Source: CAD feature listing. Evaluate the final solid. Frame: model axes, mm. A direction names the side the tool comes from. Coordinates: 2 decimals unless noted, no trailing zeros. Order: outer loops, then holes, each group sorted by start corner. A loop starts at its lowest first (then second) coordinate and runs counter-clockwise, first axis right, second up. Notation, with made-up numbers: (8.5, 27.5) -> (32.5, 27.5) arc R23 cw to (32.5, 49.5) -> close; hole circle Ø10 at (-38, 69.5). An arc over 180 degrees is marked (long way). Write item = value, one per line. Start each with the question number.
Item 1: Section query D-D (x = 8.6). Output: boundary loops of the cut face in (y, z).
Item 2: Ray query, line 1 along X through (y, z) = (3.25, -3.25); line 2 along Y through (x, z) = (3.5, 4.25); line 3 along Z through (x, y) = (5.5, 3.5). Return the intervals inside material, ascending. Write a range as [from, to].
Item 3: Mould query, pull axis X, two halves, no side actions, for faces 4 (the flat face through (3.6, -2, -7.5)), 5 (the flat face through (-18.9, -2, 5)), 6 (the flat face through (1, -3, 9)), 7 (the flat face through (-22.4, 0.5, 2.2)). Classes: released by +X, released by -X, zero draft, split by the parting line, or undercut.
Item 4: Contact query for flat-ended pins moving along their axis: pin 1 (2.5 mm diameter, centred on x = 1.5, z = -7, fed in from -Y); pin 2 (1.5 mm diameter, centred on x = -24, z = 5, fed in from +Y); pin 3 (3 mm diameter, centred on x = -8, y = 4, fed in from +Z); pin 4 (1.5 mm diameter, centred on y = -2, z = 10, fed in from -X). Output: stop coordinate, or through.
Item 5: Section query A-A (x = -12.5). Output: boundary loops of the cut face in (y, z), then the cut area to 3 significant figures.
Item 6: Set-up query: faces 1 (the flat face through (1, -1, 13)), 2 (the flat face through (-23, -1, 5)), 3 (the flat face through (-6, 3, 11.5)). Return all of +Z, -Z, +X, -X, +Y, -Y with unobstructed straight access to the full face (end or side cutting, diameter ignored); none if empty.
Item 7: Section query C-C (z = -3.5). Output: boundary loops of the cut face in (x, y), then the cut area to 3 significant figures.
Item 8: Section query B-B (y = 3.25). Output: boundary loops of the cut face in (x, z), then the cut area to 3 significant figures.
```python
from build123d import *

# Parameters (mm, degrees)
SKETCH1_W            = 33
SKETCH1_H            = 23
BOSS_EXTRUDE1_DEPTH  = 1
SKETCH2_W            = 23
SKETCH2_H            = 19
BOSS_EXTRUDE2_DEPTH  = 4
SKETCH3_W            = 8.5
SKETCH3_H            = 7
BOSS_EXTRUDE4_DEPTH  = 3
SKETCH4_R            = 1.75
BOSS_EXTRUDE5_DEPTH  = 1
SKETCH5_W            = 6
SKETCH5_H            = 6
BOSS_EXTRUDE6_DEPTH  = 0.75
SKETCH6_R            = 2.9
BOSS_EXTRUDE7_DEPTH  = 7
SKETCH7_W            = 6
SKETCH7_H            = 3
BOSS_EXTRUDE8_DEPTH  = 1.5
SKETCH8_W            = 4
SKETCH8_H            = 1
BOSS_EXTRUDE9_DEPTH  = 1
SKETCH9_W            = 3
SKETCH9_H            = 10
BOSS_EXTRUDE10_DEPTH = 4
SKETCH10_W           = 8
SKETCH10_H           = 2
BOSS_EXTRUDE11_DEPTH = 3


with BuildPart() as part:
    # Sketch1 → Boss-Extrude1 (new body)
    with BuildSketch(Plane(origin=(0, 0, 0), x_dir=(1, 0, 0), z_dir=(0, 1, 0))):
        with Locations((-5.9, -2)):
            Rectangle(SKETCH1_W, SKETCH1_H)
    extrude(amount=BOSS_EXTRUDE1_DEPTH)

    # Sketch2 → Boss-Extrude2 (add)
    with BuildSketch(Plane(origin=(0, 1, 0), x_dir=(1, 0, 0), z_dir=(0, 1, 0))):
        with Locations((-5.9, -2)):
            Rectangle(SKETCH2_W, SKETCH2_H)
    extrude(amount=BOSS_EXTRUDE2_DEPTH)

    # Sketch3 → Boss-Extrude4 (add)
    with BuildSketch(Plane(origin=(0, 0, 0), x_dir=(-1, 0, 0), z_dir=(0, -1, 0))):
        with Locations((-1.35, -9.5)):
            Rectangle(SKETCH3_W, SKETCH3_H)
    extrude(amount=BOSS_EXTRUDE4_DEPTH)

    # Sketch4 → Boss-Extrude5 (add)
    with BuildSketch(Plane.XZ):
        with Locations(Location((8.6, 11.5, 0), (0, 0, 90))):
            Circle(SKETCH4_R)
    extrude(amount=BOSS_EXTRUDE5_DEPTH)

    # Sketch5 → Boss-Extrude6 (add)
    with BuildSketch(Plane(origin=(10.6, 0, 0), x_dir=(0, 0, -1), z_dir=(1, 0, 0))):
        with Locations((3.5, 1)):
            Rectangle(SKETCH5_W, SKETCH5_H)
    extrude(amount=BOSS_EXTRUDE6_DEPTH)

    # Sketch6 → Boss-Extrude7 (add)
    with BuildSketch(Plane(origin=(11.35, 0, 0), x_dir=(0, 0, -1), z_dir=(1, 0, 0))):
        with Locations((3.5, 1)):
            Circle(SKETCH6_R)
    extrude(amount=BOSS_EXTRUDE7_DEPTH)

    # Sketch7 → Boss-Extrude8 (add)
    with BuildSketch(Plane(origin=(0, 0, 0), x_dir=(-1, 0, 0), z_dir=(0, -1, 0))):
        with Locations((-1.6, 7.5)):
            Rectangle(SKETCH7_W, SKETCH7_H)
    extrude(amount=BOSS_EXTRUDE8_DEPTH)

    # Sketch8 → Boss-Extrude9 (add)
    with BuildSketch(Plane.XZ.offset(1.5)):
        with Locations((1.6, -7.5)):
            Rectangle(SKETCH8_W, SKETCH8_H)
    extrude(amount=BOSS_EXTRUDE9_DEPTH)

    # Sketch9 → Boss-Extrude10 (add)
    with BuildSketch(Plane.XZ):
        with Locations((-20.4, 5.5)):
            Rectangle(SKETCH9_W, SKETCH9_H)
    extrude(amount=BOSS_EXTRUDE10_DEPTH)

    # Sketch10 → Boss-Extrude11 (add)
    with BuildSketch(Plane.ZY.offset(21.9)):
        with Locations((5.5, -2)):
            Rectangle(SKETCH10_W, SKETCH10_H)
    extrude(amount=BOSS_EXTRUDE11_DEPTH)


solid = part.part
```
Computed:
q1.outline = (-1, 9.75) -> (0, 9.75) -> (0, -9.5) -> (1, -9.5) -> (1, 13.5) -> (0, 13.5) -> (0, 13.25) -> (-1, 13.25) -> close
q2.line_1 = [-17.4, 5.6], [10.6, 18.35]
q2.line_2 = [0, 5]
q2.line_3 = [-7.5, 11.5]
q3.face_4 = released by +X
q3.face_5 = undercut
q3.face_6 = zero draft
q3.face_7 = released by -X
q4.pin_1 = -2.5
q4.pin_2 = -1
q4.pin_3 = 11.5
q4.pin_4 = -24.9
q5.outline = (0, -9.5) -> (1, -9.5) -> (1, -7.5) -> (5, -7.5) -> (5, 11.5) -> (1, 11.5) -> (1, 13.5) -> (0, 13.5) -> close
q5.area = 99.0 mm^2
q6.face_1 = +Z, -X, -Y
q6.face_2 = +Z, -Z, -X
q6.face_3 = +Z, +X, -X, +Y
q7.outline = (-22.4, 0) -> (10.6, 0) -> (10.6, -2) -> (11.35, -2) -> (11.35, -1.9) -> (18.35, -1.9) -> (18.35, 3.9) -> (11.35, 3.9) -> (11.35, 4) -> (10.6, 4) -> (10.6, 1) -> (5.6, 1) -> (5.6, 5) -> (-17.4, 5) -> (-17.4, 1) -> (-22.4, 1) -> close
q7.area = 170 mm^2
q8.outline = (-17.4, -7.5) -> (5.6, -7.5) -> (5.6, 11.5) -> (-17.4, 11.5) -> close; (10.6, -6.5) -> (11.35, -6.5) -> (11.35, -5.33) -> (18.35, -5.33) -> (18.35, -1.67) -> (11.35, -1.67) -> (11.35, -0.5) -> (10.6, -0.5) -> close
q8.area = 467 mm^2
